For this review, take the finished solid that the model builds, in its own axes (mm). Face numbers are marked on the shaded views. A direction names the side the tool comes from. Give positions to 0.01 mm unless a question says otherwise; leave off trailing zeros. Write each loop counter-clockwise with the first axis right and the second up, starting at its lowest first coordinate (ties: lowest second). Pieces come first, ordered by that corner, then holes.
1) We need section D-D on z = 10.5. Give the boundary of the cut face in (x, y).
2) We need section A-A on x = 0. Give the boundary of the cut face in (y, z).
3) Wall thickness on line 1 along Z through (x, y) = (8, 5); line 2 along Y through (x, z) = (7.5, 19.5); line 3 along X through (y, z) = (4, -19): over which ranges is each line inside the solid? List them lowest first.
4) We need section C-C on y = 14. Give the boundary of the cut face in (x, z), and give its area (3 significant figures).
5) We need section B-B on x = 30. Give the boundary of the cut face in (y, z), and give its area (3 significant figures).
6) For P1, Ø4, axis at x = -1.5, z = 23.5, coming from the +Y side; P2, Ø4, axis at y = 5, z = 3.5, coming from the +X side; P3, Ø2.5, axis at x = 0, y = 10.5, coming from the -Z side, all flat-tipped, find the tip position at first contact; note any pin that passes through.
7) Machinability: for the marked faces 1 and 2, which of the approach directions +Z, -Z, +X, -X, +Y, -Y give a long, thin tool a straight path to every point of the face, cutting with its end or side? Answer none if there is none.
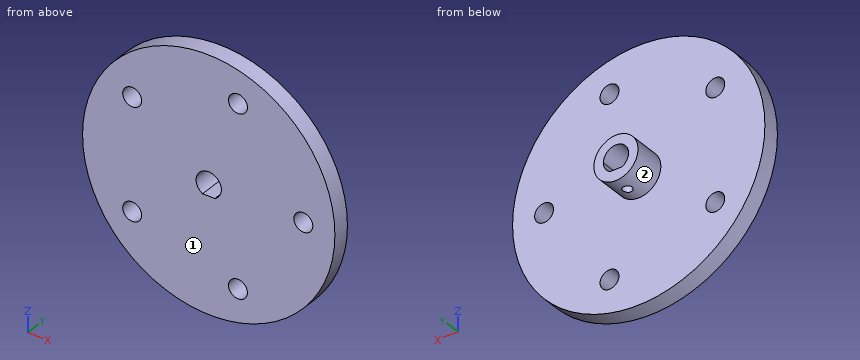
from build123d import *

# Parameters (mm, degrees)
SKETCH1_R           = 40
BOSS_EXTRUDE1_DEPTH = 5.5
SKETCH2_R           = 3
CUT_EXTRUDE1_DEPTH  = 6.5
CIRPATTERN1_COUNT   = 5
SKETCH3_R           = 7
BOSS_EXTRUDE2_DEPTH = 10
CUT_EXTRUDE2_DEPTH  = 20
SKETCH8_R           = 1.5
CUT_EXTRUDE3_DEPTH  = 10


with BuildPart() as part:
    # Sketch1 → Boss-Extrude1 (new body)
    with BuildSketch(Plane(origin=(0, 0, 0), x_dir=(1, 0, 0), z_dir=(0, 1, 0))):
        Circle(SKETCH1_R)
    extrude(amount=BOSS_EXTRUDE1_DEPTH)

    # Sketch2 → Cut-Extrude1 (cut, through all)
    with BuildSketch(Plane(origin=(0, 5.5, 0), x_dir=(1, 0, 0), z_dir=(0, 1, 0))):
        with Locations((30, 0)):
            Circle(SKETCH2_R)
    cut_extrude1 = extrude(amount=-CUT_EXTRUDE1_DEPTH, mode=Mode.SUBTRACT)

    # CirPattern1: Cut-Extrude1 ×5 about axis
    cirpattern1_axis = Axis((0, 0, 0), (0, 1, 0))
    for i in range(1, CIRPATTERN1_COUNT):
        add(cut_extrude1.rotate(cirpattern1_axis, i * 360 / CIRPATTERN1_COUNT), mode=Mode.SUBTRACT)

    # Sketch3 → Boss-Extrude2 (add)
    with BuildSketch(Plane(origin=(0, 5.5, 0), x_dir=(1, 0, 0), z_dir=(0, 1, 0))):
        Circle(SKETCH3_R)
    extrude(amount=BOSS_EXTRUDE2_DEPTH)

    # Sketch7 → Cut-Extrude2 (cut)
    with BuildSketch(Plane(origin=(0, 15.5, 0), x_dir=(1, 0, 0), z_dir=(0, 1, 0))):
        with BuildLine():
            ThreePointArc((4, 0), (3.445719569, 2.031506006), (1.936491673, 3.5))
            Line((1.936491673, 3.5), (-1.936491673, 3.5))
            ThreePointArc((-1.936491673, 3.5), (-2.031506006, -3.445719569), (4, 0))
        make_face()
    extrude(amount=-CUT_EXTRUDE2_DEPTH, mode=Mode.SUBTRACT)

    # Sketch8 → Cut-Extrude3 (cut)
    with BuildSketch(Plane.XY):
        with Locations((0, 10.5)):
            Circle(SKETCH8_R)
    extrude(amount=-CUT_EXTRUDE3_DEPTH, mode=Mode.SUBTRACT)


solid = part.part
Results list:
1. outline: (-38.6, 0) - (38.6, 0) - (38.6, 5.5) - (-38.6, 5.5) - close
2. outline: (0, -40) - (5.5, -40) - (5.5, -7) - (9, -7) - (9, -3.5) - (0, -3.5) - close; (0, 4) - (15.5, 4) - (15.5, 7) - (5.5, 7) - (5.5, 40) - (0, 40) - close; (12, -7) - (15.5, -7) - (15.5, -3.5) - (12, -3.5) - close
3. line 1: z = -39.19 to -31.25, -25.81 to 25.81, 31.25 to 39.19
3. line 2: y = 0 to 5.5
3. line 3: x = -35.2 to -26.94, -21.6 to 35.2
4. outline: circle Ø14 at (0, 0); hole (-1.94, -3.5) - (1.94, -3.5) arc R4 ccw (long way) to start
4. area: 105 mm2
5. outline: (0, -26.46) - (5.5, -26.46) - (5.5, -3) - (0, -3) - close; (0, 3) - (5.5, 3) - (5.5, 26.46) - (0, 26.46) - close
5. area: 258 mm2
6. P1: stops at y = 5.5
6. P2: stops at x = 39.97
6. P3: stops at z = 3.8
7. face 1: +Z, -Z, +X, -X, -Y
7. face 2: +Y
